Read the model definition and answer for the solid it produces. Units are mm, in the model's axes. A direction names the side the tool comes from. Round coordinates to 2 decimals unless told otherwise and drop trailing zeros. Write each loop counter-clockwise with the first axis right and the second up, starting at its lowest first coordinate (ties: lowest second). Pieces come first, ordered by that corner, then holes. Notation, with made-up numbers: (0.5, 28) -> (7.5, 28) arc R27 ccw to (7.5, 65) -> close; hole circle Ø3 at (87.25, 49). An arc over 180 degrees is marked (long way). Return JSON: item names as keys, results as strings. Group by question number.
(1) The mould has two halves that part along Y. Classify faces 4 (the flat face through (77.124, 48, 59)), 5 (the cylindrical face through (75.698, 39.922, 59.16)), 6 (the cylindrical face through (80.621, 34.844, 59.16)): released by +Y, released by -Y, zero draft, split by the parting line, or undercut.
(2) A cutting plane is placed at A-A on x = 69.5. Give the vertices of the cut face in (y, z), then the cut area to 3 significant figures.
(3) Given pin 1 (4 mm diameter, centred on x = 110, z = 88, fed in from +Y); pin 2 (3 mm diameter, centred on y = 106, z = 66.5, fed in from +X); pin 3 (4 mm diameter, centred on y = 45.5, z = 38.5, fed in from +X), each flat-ended and moving along its own axis, determine where each tip first touches the part or whether it passes through.
(4) For faces 1 (the flat face through (70, 33.418, 59)), 2 (the flat face through (5, 57, 59)), 3 (the flat face through (68, 38.418, 59)), determine the directions among +Z, -Z, +X, -X, +Y, -Y from which every point of the face is accessible in a straight line to the end or side of a thin tool.
(5) A cutting plane is placed at C-C on x = 215. Give the vertices of the cut face in (y, z).
(6) A cutting plane is placed at D-D on y = 57. Give the vertices of the cut face in (x, z), then the cut area to 3 significant figures.
(7) Straight lines are drawn through the part: line 1 (X direction, y = 40.5, z = 94.5); line 2 (Y direction, x = 67, z = 38); line 3 (X direction, y = 28, z = 24). For each, find the intervals that lie inside material, in ascending order.
```python
from build123d import *

# Parameters (mm, degrees)
BOSS_EXTRUDE1_DEPTH = 120
SKETCH3_W           = 30
SKETCH3_H           = 30
BOSS_EXTRUDE2_DEPTH = 3
SKETCH6_W           = 30.5
SKETCH6_H           = 30.5
BOSS_EXTRUDE3_DEPTH = 5.5


with BuildPart() as part:
    # Sketch1 → Boss-Extrude1 (new body)
    with BuildSketch(Plane.XY):
        with BuildLine():
            Line((2, 0), (228, 0))
            ThreePointArc((228, 0), (229.414213562, 0.585786438), (230, 2))
            Line((230, 2), (230, 3))
            ThreePointArc((230, 3), (229.414213562, 4.414213562), (228, 5))
            Line((228, 5), (10, 5))
            ThreePointArc((10, 5), (6.464466094, 6.464466094), (5, 10))
            Line((5, 10), (5, 104.939576417))
            ThreePointArc((5, 104.939576417), (6.398588401, 106.847010319), (8.638304089, 106.08672929))
            Line((8.638304089, 106.08672929), (58.028349014, 35.550435076))
            ThreePointArc((58.028349014, 35.550435076), (59.815366169, 33.983263092), (62.124109236, 33.418317258))
            Line((62.124109236, 33.418317258), (77.124109236, 33.418317258))
            ThreePointArc((77.124109236, 33.418317258), (80.659643142, 34.882783352), (82.124109236, 38.418317258))
            Line((82.124109236, 38.418317258), (82.124109236, 52.418317258))
            ThreePointArc((82.124109236, 52.418317258), (81.831216017, 53.125424039), (81.124109236, 53.418317258))
            Line((81.124109236, 53.418317258), (78.124109236, 53.418317258))
            ThreePointArc((78.124109236, 53.418317258), (77.417002454, 53.125424039), (77.124109236, 52.418317258))
            Line((77.124109236, 52.418317258), (77.124109236, 43.418317258))
            ThreePointArc((77.124109236, 43.418317258), (75.659643142, 39.882783352), (72.124109236, 38.418317258))
            Line((72.124109236, 38.418317258), (64.726944488, 38.418317258))
            ThreePointArc((64.726944488, 38.418317258), (62.418201422, 38.983263092), (60.631184267, 40.550435076))
            Line((60.631184267, 40.550435076), (5.597169987, 119.147152873))
            ThreePointArc((5.597169987, 119.147152873), (4.882363125, 119.774021666), (3.958865899, 120))
            Line((3.958865899, 120), (2, 120))
            ThreePointArc((2, 120), (0.585786438, 119.414213562), (0, 118))
            Line((0, 118), (0, 2))
            ThreePointArc((0, 2), (0.585786438, 0.585786438), (2, 0))
        make_face()
    extrude(amount=BOSS_EXTRUDE1_DEPTH)

    # Sketch3 → Boss-Extrude2 (add)
    with BuildSketch(Plane(origin=(0, 0, 0), x_dir=(1, 0, 0), z_dir=(0, 1, 0))):
        with Locations((205, -60)):
            Rectangle(SKETCH3_W, SKETCH3_H)
    extrude(amount=BOSS_EXTRUDE2_DEPTH)

    # Sketch6 → Boss-Extrude3 (add)
    with BuildSketch(Plane(origin=(0, 0, 0), x_dir=(1, 0, 0), z_dir=(0, 1, 0))):
        with Locations((206.124109236, -60)):
            Rectangle(SKETCH6_W, SKETCH6_H)
    extrude(amount=BOSS_EXTRUDE3_DEPTH)


solid = part.part
```
Checks:
{
 "1": {"face 4": "zero draft", "face 5": "released by +Y", "face 6": "undercut"},
 "2": {"outline": "(0, 0) -> (5, 0) -> (5, 120) -> (0, 120) -> close; (33.42, 0) -> (38.42, 0) -> (38.42, 120) -> (33.42, 120) -> close", "area": "1,200 mm^2"},
 "3": {"pin 1": "stops at y = 5", "pin 2": "stops at x = 15.85", "pin 3": "stops at x = 82.12"},
 "4": {"face 1": "+Z, -Z, +X", "face 2": "+Z, -Z", "face 3": "+Z, -Z, +Y"},
 "5": {"outline": "(0, 0) -> (5, 0) -> (5, 44.75) -> (5.5, 44.75) -> (5.5, 75.25) -> (5, 75.25) -> (5, 120) -> (0, 120) -> close"},
 "6": {"outline": "(0, 0) -> (5, 0) -> (5, 120) -> (0, 120) -> close; (43.01, 0) -> (49.11, 0) -> (49.11, 120) -> (43.01, 120) -> close", "area": "1,330 mm^2"},
 "7": {"line 1": "x = 0 to 5, 54.56 to 60.67, 76.18 to 82.12", "line 2": "y = 0 to 5, 33.42 to 38.42", "line 3": "x = 0 to 5"}
}
